Design review of the part built by this model. Coordinates are the model's own, in mm. Give positions to 0.01 mm unless a question says otherwise; leave off trailing zeros. Write each loop counter-clockwise with the first axis right and the second up, starting at its lowest first coordinate (ties: lowest second). Pieces come first, ordered by that corner, then holes.
```python
from build123d import *

# Parameters (mm, degrees)
SKETCH1_R           = 2.1828125
BOSS_EXTRUDE1_DEPTH = 3.175
CHAMFER1_SIZE       = 0.396875


with BuildPart() as part:
    # Sketch1 → Boss-Extrude1 (new body, symmetric)
    with BuildSketch(Plane(origin=(0, 0, 0), x_dir=(1, 0, 0), z_dir=(0, 1, 0))):
        with BuildLine():
            Line((-25.4, -19.05), (-25.4, -31.75))
            ThreePointArc((-25.4, -31.75), (-20.745028245, -37.869589794), (-13.604919922, -35.017048047))
            Line((-13.604919922, -35.017048047), (4.519073196, -4.810392851))
            ThreePointArc((4.519073196, -4.810392851), (4.841622185, -4.365295225), (5.236106863, -3.98250078))
            Line((5.236106863, -3.98250078), (29.411012744, 15.71466781))
            ThreePointArc((29.411012744, 15.71466781), (30.992963694, 23.644368325), (23.505953794, 26.698447861))
            Line((23.505953794, 26.698447861), (-1.894046206, 18.760947861))
            ThreePointArc((-1.894046206, 18.760947861), (-3.926469495, 17.690524752), (-5.445080078, 15.967048047))
            Line((-5.445080078, 15.967048047), (-24.495080078, -15.782951953))
            ThreePointArc((-24.495080078, -15.782951953), (-25.169589794, -17.354971755), (-25.4, -19.05))
        make_face()
        Circle(SKETCH1_R, mode=Mode.SUBTRACT)
        with Locations((0, 12.7)):
            Circle(SKETCH1_R, mode=Mode.SUBTRACT)
        with Locations((-19.05, -19.05)):
            Circle(SKETCH1_R, mode=Mode.SUBTRACT)
        with Locations((-19.05, -31.75)):
            Circle(SKETCH1_R, mode=Mode.SUBTRACT)
        with Locations((25.4, 20.6375)):
            Circle(SKETCH1_R, mode=Mode.SUBTRACT)
    extrude(amount=BOSS_EXTRUDE1_DEPTH, both=True)

    # Chamfer1
    chamfer1_edges = [part.edges().sort_by_distance(p)[0] for p in [
        (-4.542923363, -3.175, 19.913720449),
        (-20.745028245, -3.175, 37.869589794),
        (-25.4, -3.175, 25.4),
        (-25.169589794, -3.175, 17.354971755),
        (-14.970080078, -3.175, -0.092048047),
        (-3.926469495, -3.175, -17.690524752),
        (10.805953794, -3.175, -22.729697861),
        (30.992963694, 3.175, -23.644368325),
        (30.992963694, -3.175, -23.644368325),
        (17.323559803, -3.175, -5.866083515),
        (4.841622185, -3.175, 4.365295225),
        (10.805953794, 3.175, -22.729697861),
        (-3.926469495, 3.175, -17.690524752),
        (-14.970080078, 3.175, -0.092048047),
        (-2.1828125, -3.175, 0),
        (-2.1828125, 3.175, 0),
        (-25.169589794, 3.175, 17.354971755),
        (-2.1828125, -3.175, -12.7),
        (-2.1828125, 3.175, -12.7),
        (-25.4, 3.175, 25.4),
        (-21.2328125, -3.175, 19.05),
        (-21.2328125, 3.175, 19.05),
        (-20.745028245, 3.175, 37.869589794),
        (-21.2328125, -3.175, 31.75),
        (-21.2328125, 3.175, 31.75),
        (-4.542923363, 3.175, 19.913720449),
        (23.2171875, -3.175, -20.6375),
        (23.2171875, 3.175, -20.6375),
        (4.841622185, 3.175, 4.365295225),
        (17.323559803, 3.175, -5.866083515),
    ]]
    chamfer(chamfer1_edges, length=CHAMFER1_SIZE)


solid = part.part
```
(1) To check wall thickness, follow L1, parallel to Z at x = 1.5, y = 1; L2, parallel to Z at x = -19.05, y = 0.95; L3, parallel to X at y = 0.8, z = 31.75. State the ranges of each line that lie inside material, in increasing order.
Resolved:
L1: z = -19.82 to -14.29, -11.11 to -1.59, 1.59 to 9.84
L2: z = 6.71 to 16.87, 21.23 to 29.57, 33.93 to 38.1
L3: x = -25.4 to -21.23, -16.87 to -11.64
(2) Mouldability with a two-part tool opening along Z and no side actions: class faces 1 (the face through (-1.73, -0.04, 1.33)), 2 (the face through (-14.84, 0.04, -0.31)), 3 (the face through (17.027, -2.979, -5.884)) as pulls with the +Z half, pulls with the -Z half, needs draft (parallel to the pull), parting line crosses it, or undercut.
Resolved:
face 1: undercut
face 2: pulls with the -Z half
face 3: pulls with the +Z half
(3) Consider section B-B, the plane z = 0. Give the boundary of the cut face in (x, y) (3 decimals).
Resolved:
outline: (-15.025, -2.778) - (-14.562, -3.175) - (-2.58, -3.175) - (-2.183, -2.778) - (-2.183, 2.778) - (-2.58, 3.175) - (-14.562, 3.175) - (-15.025, 2.778) - close; (2.183, -2.778) - (2.58, -3.175) - (9.496, -3.175) - (10.124, -2.778) - (10.124, 2.778) - (9.496, 3.175) - (2.58, 3.175) - (2.183, 2.778) - close
(4) Consider section C-C, the plane y = 2. Give the number of separate pieces and of enclosed holes in the cut face, then the cut area to 3 significant figures.
Resolved:
separate pieces: 1
enclosed holes: 5
area: 1,380 mm2
(5) Consider section D-D, the plane x = -19.05. Give the boundary of the cut face in (y, z) (3 decimals), then the cut area to 3 significant figures.
Resolved:
outline: (-3.175, 7.479) - (-2.778, 6.708) - (2.778, 6.708) - (3.175, 7.479) - (3.175, 16.47) - (2.778, 16.867) - (-2.778, 16.867) - (-3.175, 16.47) - close; (-3.175, 21.63) - (-2.778, 21.233) - (2.778, 21.233) - (3.175, 21.63) - (3.175, 29.17) - (2.778, 29.567) - (-2.778, 29.567) - (-3.175, 29.17) - close; (-3.175, 34.33) - (-2.778, 33.933) - (2.778, 33.933) - (3.175, 34.33) - (3.175, 37.703) - (2.778, 38.1) - (-2.778, 38.1) - (-3.175, 37.703) - close
area: 143 mm2
(6) Clearance check with flat-ended pins moving along their axes: P1, Ø1, axis at x = 24, y = 0, coming from the +Z side; P2, Ø5, axis at x = -19.05, z = 31.75, coming from the -Y side. State where each tip first meets the part, or that it passes through.
Resolved:
P1: stops at z = -10.9
P2: stops at y = -3.1
(7) Consider section A-A, the plane x = 0. Give the boundary of the cut face in (y, z) (3 decimals).
Resolved:
outline: (-3.175, -18.937) - (-2.778, -19.353) - (2.778, -19.353) - (3.175, -18.937) - (3.175, -15.28) - (2.778, -14.883) - (-2.778, -14.883) - (-3.175, -15.28) - close; (-3.175, -10.12) - (-2.778, -10.517) - (2.778, -10.517) - (3.175, -10.12) - (3.175, -2.58) - (2.778, -2.183) - (-2.778, -2.183) - (-3.175, -2.58) - close; (-3.175, 2.58) - (-2.778, 2.183) - (2.778, 2.183) - (3.175, 2.58) - (3.175, 11.571) - (2.778, 12.342) - (-2.778, 12.342) - (-3.175, 11.571) - close
